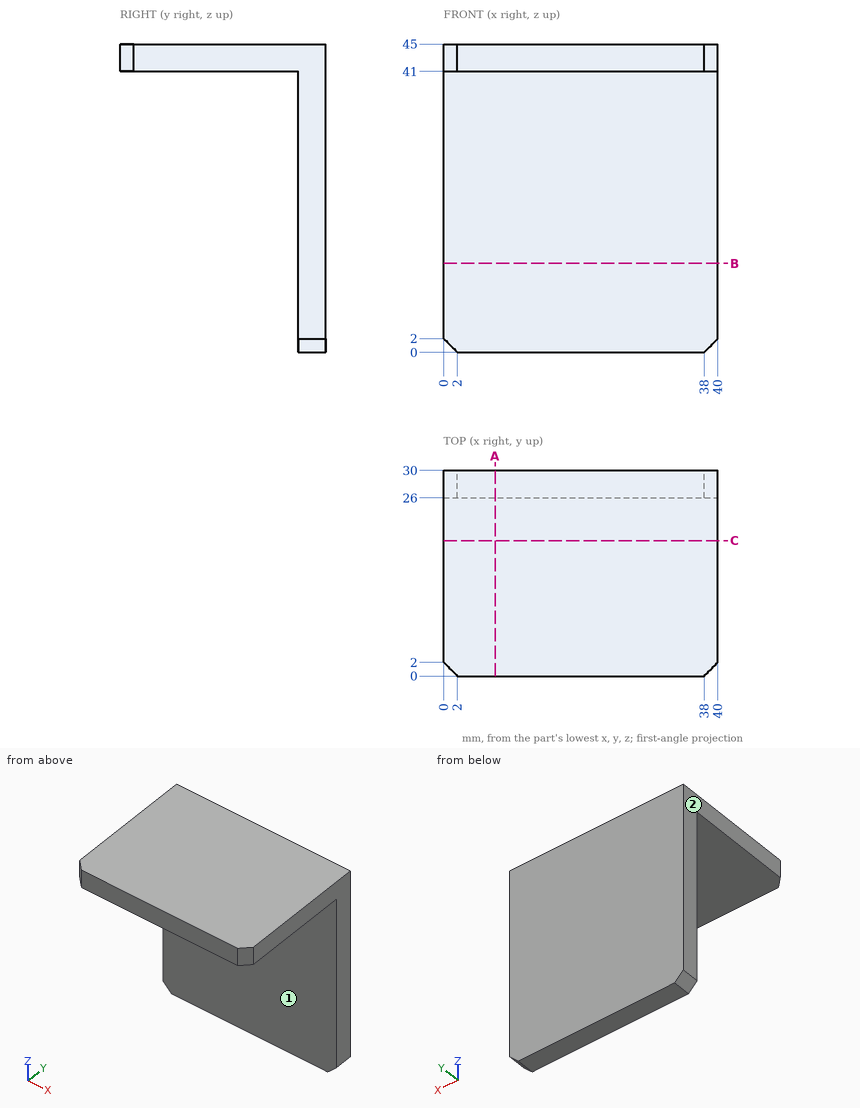
Check sheet for the drawn part. Datum: minimum x, y, z corner. Units: mm. A direction names the side the tool comes from. Give positions to 0.01 mm unless a question says otherwise; leave off trailing zeros. Loops run counter-clockwise (first coordinate to the right, second up) from the corner with the lowest first, then second, coordinate; pieces in that order, holes last. Notation, with made-up numbers: M 52,80 L 60,80 A37 ccw 60,119 Z; hole C 78,47 d4. An arc over 180 degrees is marked long. Answer as CSV lines item,"result".
Item 1: Sectioned sample at C-C, the plane y = 19.75. Enter the section's corners in (x, z).
Reply:
outline,"M 0,41 L 40,41 L 40,45 L 0,45 Z"
Item 2: Scan lines: L1, parallel to Y at x = 24, z = 6.5; L2, parallel to Z at x = 33, y = 5.75. Record each from-to range of solid material in increasing order.
Reply:
L1,"26 to 30"
L2,"41 to 45"
Item 3: Sectioned sample at B-B, the plane z = 13. Enter the section's corners in (x, y).
Reply:
outline,"M 0,26 L 40,26 L 40,30 L 0,30 Z"
Item 4: Sectioned sample at A-A, the plane x = 7.5. Enter the section's corners in (y, z).
Reply:
outline,"M 0,41 L 26,41 L 26,0 L 30,0 L 30,45 L 0,45 Z"
Item 5: Set-up check for the marked faces 1 and 2: record each of +Z, -Z, +X, -X, +Y, -Y from which the full face is reachable in a straight line by a thin tool's end or side.
Reply:
face 1,"-Z, +X, -X, -Y"
face 2,"+Z, -Z, -X, +Y, -Y"
Item 6: Depth check by flat-ended pin: pin 1 Ø12 at (x, y) = (32.5, 19.5) entering from -Z; pin 2 Ø1.5 at (x, z) = (8.5, 9.5) entering from -Y. Enter the tip coordinate at first touch or a pass-through.
Reply:
pin 1,"z = 41"
pin 2,"y = 26"
